```python
from build123d import *

# Parameters (mm, degrees)
SKETCH1_W            = 30
SKETCH1_H            = 5.5
BOSS_EXTRUDE1_DEPTH  = 25
BOSS_EXTRUDE3_DEPTH  = 100
SKETCH5_R            = 0.2875
BOSS_EXTRUDE9_DEPTH  = 1
SKETCH5_10_W         = 17.4
SKETCH5_10_H         = 1
CUT_EXTRUDE1_DEPTH   = 3
SKETCH1_5_W          = 30
SKETCH1_5_H          = 5.5
BOSS_EXTRUDE11_DEPTH = 15


with BuildPart() as part:
    # Sketch1 → Boss-Extrude1 (new body)
    with BuildSketch(Plane.XY):
        with Locations((-15, 2.75)):
            Rectangle(SKETCH1_W, SKETCH1_H)
    extrude(amount=-BOSS_EXTRUDE1_DEPTH)

    # Sketch3 → Boss-Extrude3 (add)
    with BuildSketch(Plane(origin=(0, 0, -25), x_dir=(-1, 0, 0), z_dir=(0, 0, -1))):
        with BuildLine():
            ThreePointArc((29, 2.5), (27, 4.5), (25, 2.5))
            Line((25, 2.5), (26.984705643, 2.5))
            Line((26.984705643, 2.5), (26.984705643, 0.50005848))
            ThreePointArc((26.984705643, 0.50005848), (28.408795813, 1.080389364), (29, 2.5))
        make_face()
        with BuildLine():
            Line((26.984705643, 2.5), (25, 2.5))
            ThreePointArc((25, 2.5), (25.580389364, 1.091204187), (26.984705643, 0.50005848))
            Line((26.984705643, 0.50005848), (26.984705643, 2.5))
        make_face()
        with BuildLine():
            Line((25, 2.5), (5, 2.5))
            ThreePointArc((5, 2.5), (4.414213562, 1.085786438), (3, 0.5))
            Line((3, 0.5), (3, 0))
            Line((3, 0), (26.984705643, 0))
            Line((26.984705643, 0), (26.984705643, 0.50005848))
            ThreePointArc((26.984705643, 0.50005848), (25.580389364, 1.091204187), (25, 2.5))
        make_face()
        with BuildLine():
            Line((3, 0.5), (3, 2.5))
            Line((3, 2.5), (5, 2.5))
            ThreePointArc((5, 2.5), (1.585786438, 3.914213562), (3, 0.5))
        make_face()
        with BuildLine():
            Line((5, 2.5), (3, 2.5))
            Line((3, 2.5), (3, 0.5))
            ThreePointArc((3, 0.5), (4.414213562, 1.085786438), (5, 2.5))
        make_face()
    extrude(amount=BOSS_EXTRUDE3_DEPTH)

    # Sketch5 → Boss-Extrude9 (add)
    with BuildSketch(Plane(origin=(0, 5.5, 0), x_dir=(1, 0, 0), z_dir=(0, 1, 0))):
        Polygon((-6.3, 24), (-6.3, 21), (-13.1, 21), (-13.1, 0), (0, 0), (0, 25), (-6.3, 25), align=None)
        Polygon((-16.9, 0), (-16.9, 21), (-23.7, 21), (-23.7, 24), (-23.7, 25), (-30, 25), (-30, 0), align=None)
        with Locations(Location((-23.0875, 21.7125, 0), (0, 0, 180))):
            Circle(SKETCH5_R)
        with Locations(Location((-23.0875, 23.2875, 0), (0, 0, 180))):
            Circle(SKETCH5_R)
        with Locations(Location((-6.9125, 23.2875, 0), (0, 0, 180))):
            Circle(SKETCH5_R)
        with Locations(Location((-6.9125, 21.7125, 0), (0, 0, 180))):
            Circle(SKETCH5_R)
    extrude(amount=BOSS_EXTRUDE9_DEPTH)

    # Sketch5_10 → Cut-Extrude1 (cut)
    with BuildSketch(Plane(origin=(0, 5.5, 0), x_dir=(1, 0, 0), z_dir=(0, 1, 0))):
        with Locations((-15, 24.5)):
            Rectangle(SKETCH5_10_W, SKETCH5_10_H)
    extrude(amount=-CUT_EXTRUDE1_DEPTH, mode=Mode.SUBTRACT)

    # Sketch1_5 → Boss-Extrude11 (add)
    with BuildSketch(Plane.XY):
        with Locations((-15, 2.75)):
            Rectangle(SKETCH1_5_W, SKETCH1_5_H)
    extrude(amount=BOSS_EXTRUDE11_DEPTH)


solid = part.part
```
Geometry: final body of the model. Coordinates: model frame, mm. A direction names the side the tool comes from. Round coordinates to 2 decimals unless told otherwise and drop trailing zeros. Order: outer loops, then holes, each group sorted by start corner. A loop starts at its lowest first (then second) coordinate and runs counter-clockwise, first axis right, second up. Notation, with made-up numbers: (13, -21) -> (49, -21) arc R18 ccw to (49, -16) -> close; hole circle Ø3 at (85.25, 29). An arc over 180 degrees is marked (long way). Use CSV: the item, a comma, the result in double quotes. Start each with the question number.
1) Section A-A (z = -39.5). Return the cut outline in (x, y), and give its area (3 significant figures).
2) Set-up query: faces 1 (the face through (-6.3, 6, -24)), 2 (the face through (0, 3, -5)), 3 (the face through (-1.633, 3.96, -74.3)). Return all of +Z, -Z, +X, -X, +Y, -Y with unobstructed straight access to the full face (end or side cutting, diameter ignored); none if empty.
3) First-contact query: pin 1 Ø1.5 at (x, y) = (-14, 4) entering from -Z; pin 2 Ø0.8 at (y, z) = (6, -15) entering from +X; pin 3 Ø0.5 at (x, y) = (-9, 6) entering from +Z; pin 4 Ø0.6 at (y, z) = (0, -98.5) entering from +X. Flat tips, straight axial feed; report the tip coordinate or a pass-through.
4) Draft query along X for faces 4 (the face through (-15, 3, 15)), 5 (the face through (-30, 3, -5)), 6 (the face through (-23.7, 5.4, -24.3)). Return one class per face: +X half, -X half, draft (parallel to the pull), parting line (faces both ways), or undercut.
5) Material intervals for line 1 along Y through (x, z) = (-5.5, -91.5); line 2 along Z through (x, y) = (-4, 6); line 3 along X through (y, z) = (3.75, -96.5), sorted ascending. Write a range as from..to.
Returned:
1,outline,"(-26.98, 0) -> (-3, 0) -> (-3, 0.5) arc R2 ccw (long way) to (-5, 2.5) -> (-25, 2.5) arc R2 ccw (long way) to (-26.98, 0.5) -> close"
1,area,"78.8 mm²"
2,face 1,"-Z, +Y"
2,face 2,"+Z, -Z, +X, +Y, -Y"
2,face 3,"-Z"
3,pin 1,"stops at z = -24"
3,pin 2,"stops at x = 0"
3,pin 3,"stops at z = 0"
3,pin 4,"stops at x = -3"
4,face 4,"draft"
4,face 5,"-X half"
4,face 6,"undercut"
5,line 1,"y = 0..2.5"
5,line 2,"z = -25..0"
5,line 3,"x = -28.56..-25.44, -4.56..-1.44"
